Design review of the part built by this model. Coordinates are the model's own, in mm. Round coordinates to 2 decimals unless told otherwise and drop trailing zeros. Loops run counter-clockwise (first coordinate to the right, second up) from the corner with the lowest first, then second, coordinate; pieces in that order, holes last. Notation, with made-up numbers: (6, 63) -> (56, 63) arc R18 ccw to (56, 95) -> close; hole circle Ø5 at (-20, 78). An arc over 180 degrees is marked (long way). Use a Markdown table: item, result. Add a question column.
from build123d import *

# Parameters (mm, degrees)
F1_DEPTH = 6.35
F2_D     = 17.5
F3_D     = 6.35
F4_D     = 22.5


with BuildPart() as f1:
    # F0 (on Top) → F1 (new body)
    with BuildSketch(Plane.XY):
        Polygon((38.1, 65.9911357684), (-31.75, 65.9911357684), (-66.675, 5.499261314), (-31.75, -54.9926131403), (38.1, -54.9926131403), (73.025, 5.499261314), align=None)
    extrude(amount=F1_DEPTH)

    # F2 (through all)
    with Locations(Plane(origin=(0, 0, 0), x_dir=(1, 0, 0), z_dir=(0, 0, -1))):
        with Locations((25.195854684, -44.1132237642), (47.625, -5.499261314), (25.195854684, 33.1147011361), (-18.845854684, 33.1147011361), (-41.275, -5.499261314), (-18.5662683496, -44.2805572462)):
            Hole(F2_D / 2)

    # F3 (through all)
    with Locations(Plane(origin=(0, 0, 0), x_dir=(1, 0, 0), z_dir=(0, 0, -1))):
        with Locations((64.135, -5.499261314), (-27.2335491394, 47.3353439388), (-27.2335491394, -58.3338665669)):
            Hole(F3_D / 2)

    # F4 (through all)
    with Locations(Plane(origin=(0, 0, 0), x_dir=(1, 0, 0), z_dir=(0, 0, -1))):
        with Locations((3.175, -5.499261314)):
            Hole(F4_D / 2)


solid = f1.part
1. Consider section A-A on x = 52.5. State the section outline as (y, z) points, plus the area to 3 significant figures.
2. To check wall thickness, follow probe 1 along Y at (x, z) = (-19, 2.25); probe 2 along X at (y, z) = (-32, 5); probe 3 along Y at (x, z) = (-29, 5.25). State the ranges of each line that lie inside material, in increasing order. Write a range as from..to.
3. Consider section C-C on z = 2.5. Give the number of separate pieces and of enclosed holes in the cut face, plus the area to 3 significant figures.
4. Consider section D-D on x = -1. State the section outline as (y, z) points.
5. Mouldability with a two-part tool opening along Y and no side actions: class faces 1 (the face through (18, 6, 0)), 2 (the face through (-48.968, 36.169, 3.131)), 3 (the face through (42.92, -1.88, 3.22)), 4 (the face through (55.3, -25.2, 3.1)) as +Y half, -Y half, draft (parallel to the pull), parting line (faces both ways), or undercut.
6. Consider section B-B on y = 51. State the section outline as (x, z) points, plus the area to 3 significant figures.
7. Insertion check: P1, Ø1, axis at y = -40.5, z = 4, coming from the +X side; P2, Ø3, axis at y = -9.5, z = 5.5, coming from the -X side. Each pin has a flat end and moves straight along its axis. Give the tip position at first contact, or say it passes through.
Verdict:
| question | item | result |
|---|---|---|
| 1 | outline | (-30.05, 0) -> (-1.77, 0) -> (-1.77, 6.35) -> (-30.05, 6.35) -> close; (12.77, 0) -> (41.05, 0) -> (41.05, 6.35) -> (12.77, 6.35) -> close |
| 1 | area | 359 mm² |
| 2 | probe 1 | y = -54.99..-41.86, -24.37..35.54, 53.02..65.99 |
| 2 | probe 2 | x = -45.02..-27.52, -10.17..16.52, 33.87..51.37 |
| 2 | probe 3 | y = -54.99..-49.97, -44.7..55.7, 60.97..65.99 |
| 3 | separate pieces | 1 |
| 3 | enclosed holes | 10 |
| 3 | area | 10,700 mm² |
| 4 | outline | (-54.99, 0) -> (-4.95, 0) -> (-4.95, 6.35) -> (-54.99, 6.35) -> close; (15.95, 0) -> (65.99, 0) -> (65.99, 6.35) -> (15.95, 6.35) -> close |
| 5 | face 1 | draft |
| 5 | face 2 | +Y half |
| 5 | face 3 | undercut |
| 5 | face 4 | -Y half |
| 6 | outline | (-40.41, 0) -> (-24.17, 0) -> (-24.17, 6.35) -> (-40.41, 6.35) -> close; (-12.96, 0) -> (19.8, 0) -> (19.8, 6.35) -> (-12.96, 6.35) -> close; (30.59, 0) -> (46.76, 0) -> (46.76, 6.35) -> (30.59, 6.35) -> close |
| 6 | area | 414 mm² |
| 7 | P1 | stops at x = 46.76 |
| 7 | P2 | stops at x = -58.88 |
